from build123d import *

# Parameters (mm, degrees)
F1_DEPTH = 4


with BuildPart() as f1:
    # F0 (on Front) → F1 (new body)
    with BuildSketch(Plane.XZ):
        with BuildLine():
            Line((15.75, 0), (4, 0))
            ThreePointArc((4, 0), (2.828427, -2.828427), (0, -4))
            Line((0, -4), (0, -13.5))
            Line((0, -13.5), (24, -13.5))
            Line((24, -13.5), (24, 0))
            Line((24, 0), (20.75, 0))
            ThreePointArc((20.75, 0), (18.25, -2.5), (15.75, 0))
        make_face()
        with BuildLine():
            ThreePointArc((0, 4), (2.828427, 2.828427), (4, 0))
            Line((4, 0), (15.75, 0))
            ThreePointArc((15.75, 0), (18.25, 2.5), (20.75, 0))
            Line((20.75, 0), (24, 0))
            Line((24, 0), (24, 13.5))
            Line((24, 13.5), (0, 13.5))
            Line((0, 13.5), (0, 4))
        make_face()
        with BuildLine():
            ThreePointArc((-4, 0), (-2.828427, 2.828427), (0, 4))
            Line((0, 4), (0, 13.5))
            Line((0, 13.5), (-24, 13.5))
            Line((-24, 13.5), (-24, 0))
            Line((-24, 0), (-20.75, 0))
            ThreePointArc((-20.75, 0), (-18.25, 2.5), (-15.75, 0))
            Line((-15.75, 0), (-4, 0))
        make_face()
        with BuildLine():
            Line((0, -13.5), (0, -4))
            ThreePointArc((0, -4), (-2.828427, -2.828427), (-4, 0))
            Line((-4, 0), (-15.75, 0))
            ThreePointArc((-15.75, 0), (-18.25, -2.5), (-20.75, 0))
            Line((-20.75, 0), (-24, 0))
            Line((-24, 0), (-24, -13.5))
            Line((-24, -13.5), (0, -13.5))
        make_face()
    extrude(amount=F1_DEPTH)


solid = f1.part
Could you check a few things on this model? Use its own coordinates, in mm. Round coordinates to 2 decimals unless told otherwise and drop trailing zeros. Write each loop counter-clockwise with the first axis right and the second up, starting at its lowest first coordinate (ties: lowest second). Pieces come first, ordered by that corner, then holes. Notation, with made-up numbers: (-16, 9.5) -> (41, 9.5) arc R30 cw to (41, 44.5) -> close; hole circle Ø6 at (55, 79.25). An arc over 180 degrees is marked (long way). Use a Markdown table: item, result.
1. Please list where these lines run through material, in increasing order: probe 1 along Z at (x, y) = (18.25, -1.3); probe 2 along X at (y, z) = (-0.25, 0.5); probe 3 along Z at (x, y) = (20, -3.3).
Answer key:
| item | result |
|---|---|
| probe 1 | z = -13.5 to -2.5, 2.5 to 13.5 |
| probe 2 | x = -24 to -20.7, -15.8 to -3.97, 3.97 to 15.8, 20.7 to 24 |
| probe 3 | z = -13.5 to -1.79, 1.79 to 13.5 |
2. If we section it at A-A (x = -18.25): List the corners of the cut face in (y, z) for me, then the cut area to 3 significant figures.
Answer key:
| item | result |
|---|---|
| outline | (-4, -13.5) -> (0, -13.5) -> (0, -2.5) -> (-4, -2.5) -> close; (-4, 2.5) -> (0, 2.5) -> (0, 13.5) -> (-4, 13.5) -> close |
| area | 88.0 mm^2 |
3. If we section it at C-C (x = 2): List the corners of the cut face in (y, z) for me.
Answer key:
| item | result |
|---|---|
| outline | (-4, -13.5) -> (0, -13.5) -> (0, -3.46) -> (-4, -3.46) -> close; (-4, 3.46) -> (0, 3.46) -> (0, 13.5) -> (-4, 13.5) -> close |
4. If we section it at B-B (y = -1): List the corners of the cut face in (x, z) for me, then the cut area to 3 significant figures.
Answer key:
| item | result |
|---|---|
| outline | (-24, -13.5) -> (24, -13.5) -> (24, 13.5) -> (-24, 13.5) -> close; hole circle Ø5 at (-18.25, 0); hole circle Ø8 at (0, 0); hole circle Ø5 at (18.25, 0) |
| area | 1,210 mm^2 |
5. We'd pull the mould along X, two halves only. Please class faces 1 (the face through (24, -2, 0)), 2 (the face through (5, 0, 0)), 3 (the face through (-20.748, -1.972, -0.11)): +X half, -X half, draft (parallel to the pull), parting line (faces both ways), or undercut.
Answer key:
| item | result |
|---|---|
| face 1 | +X half |
| face 2 | draft |
| face 3 | undercut |
